Part model, mm, in its own coordinate system. Face numbers are marked on the shaded views. A direction names the side the tool comes from. Give positions to 0.01 mm unless a question says otherwise; leave off trailing zeros. Order: outer loops, then holes, each group sorted by start corner. A loop starts at its lowest first (then second) coordinate and runs counter-clockwise, first axis right, second up.
from build123d import *

# Parameters (mm, degrees)
AUFSATZ_LINEAR_AUSTRAGEN1_DEPTH = 200
AUFSATZ_LINEAR_AUSTRAGEN2_DEPTH = 10
SPIEGELN2_DEPTH                 = 96.337442911
SPIEGELN2_START                 = 104.471237307
SPIEGELN2_2_DEPTH               = 95.528762693
SPIEGELN2_START_2               = 96.337442911
SPIEGELN2_3_DEPTH               = 8.133794396


with BuildPart() as part:
    # Skizze1 → Aufsatz-Linear austragen1 (new body)
    with BuildSketch(Plane.XY):
        with BuildLine():
            Line((0, 38), (-1.4223e-13, 597.0183631567951))
            Line((-1.4223e-13, 597.0183631567951), (125, 597.0183631567951))
            Line((125, 597.0183631567951), (125, 183.98587038126252))
            Line((125, 183.98587038126252), (25.100000000000005, 10.953994705129267))
            ThreePointArc((25.100000000000005, 10.953994705129267), (19.930243299860727, 6.526867548832285), (18.000000000000007, -3.47e-15))
            Line((18.000000000000007, -3.47e-15), (18.000000000000007, -75))
            Line((18.000000000000007, -75), (0, -75))
            Line((0, -75), (0, -38.000000000000014))
            Line((0, -38.000000000000014), (10.000000000000002, -23.000000000000014))
            Line((10.000000000000002, -23.000000000000014), (10.000000000000007, -1.388e-14))
            Line((10.000000000000007, -1.388e-14), (10.000000000000002, 22.999999999999986))
            Line((10.000000000000002, 22.999999999999986), (0, 38))
        make_face()
    extrude(amount=AUFSATZ_LINEAR_AUSTRAGEN1_DEPTH)

    # Skizze2 → Aufsatz-Linear austragen2 (add)
    with BuildSketch(Plane(origin=(0, 597.0183631567951, 0), x_dir=(1, 0, 0), z_dir=(0, 1, 0))):
        Polygon((-1.4223e-13, -200), (35.99999999999986, -200), (35.999999999999865, 0), (1.225e-14, 0), align=None)
    extrude(amount=AUFSATZ_LINEAR_AUSTRAGEN2_DEPTH)

    # Skizze3 → Schnitt-Rotation1 (revolve, cut)
    with BuildSketch(Plane(origin=(0, 0, 0), x_dir=(0, 0, -1), z_dir=(1, 0, 0))):
        Polygon((-105.00000000000001, 72.00000000000001), (-107.50000000000001, 69.5), (-107.50000000000001, 0), (-100, 0), (-100, 72.00000000000001), (-100, 74.88675134594817), align=None)
    revolve(axis=Axis((0, 0, 100), (0, 1, 0)), mode=Mode.SUBTRACT)

    # Spiegeln2: read off the stored shape, not the designer's step
    # Spiegeln2 outline → Spiegeln2 (add)
    with BuildSketch(Plane.XY):
        with BuildLine():
            Line((-36, 607.018363157), (-36, 597.018363157))
            Line((-36, 597.018363157), (-125, 597.018363157))
            Line((-125, 597.018363157), (-125, 183.985870381))
            Line((-125, 183.985870381), (-25.1, 10.953994705))
            ThreePointArc((-25.1, 10.953994705), (-19.9302433, 6.526867549), (-18, 0))
            Line((-18, 0), (-18, -75))
            Line((-18, -75), (0, -75))
            Line((0, -75), (0, -38))
            Line((0, -38), (-10, -23))
            Line((-10, -23), (-10, 23))
            Line((-10, 23), (0, 38))
            Line((0, 38), (0, 607.018363157))
            Line((0, 607.018363157), (-36, 607.018363157))
        make_face()
    extrude(amount=SPIEGELN2_DEPTH)

    # Spiegeln2 2 outline → Spiegeln2 2 (add)
    with BuildSketch(Plane.XY.offset(SPIEGELN2_START)):
        with BuildLine():
            Line((-36, 607.018363157), (-36, 597.018363157))
            Line((-36, 597.018363157), (-125, 597.018363157))
            Line((-125, 597.018363157), (-125, 183.985870381))
            Line((-125, 183.985870381), (-25.1, 10.953994705))
            ThreePointArc((-25.1, 10.953994705), (-19.9302433, 6.526867549), (-18, 0))
            Line((-18, 0), (-18, -75))
            Line((-18, -75), (0, -75))
            Line((0, -75), (0, -38))
            Line((0, -38), (-10, -23))
            Line((-10, -23), (-10, 23))
            Line((-10, 23), (0, 38))
            Line((0, 38), (0, 607.018363157))
            Line((0, 607.018363157), (-36, 607.018363157))
        make_face()
    extrude(amount=SPIEGELN2_2_DEPTH)

    # Spiegeln2 3 outline → Spiegeln2 3 (add)
    with BuildSketch(Plane.XY.offset(SPIEGELN2_START_2)):
        with BuildLine():
            Line((-36, 607.018363157), (-36, 597.018363157))
            Line((-36, 597.018363157), (-125, 597.018363157))
            Line((-125, 597.018363157), (-125, 183.985870381))
            Line((-125, 183.985870381), (-25.1, 10.953994705))
            ThreePointArc((-25.1, 10.953994705), (-19.9302433, 6.526867549), (-18, 0))
            Line((-18, 0), (-18, -75))
            Line((-18, -75), (0, -75))
            Line((0, -75), (0, -38))
            Line((0, -38), (-10, -23))
            Line((-10, -23), (-10, 23))
            Line((-10, 23), (0, 38))
            Line((0, 38), (0, 607.018363157))
            Line((0, 607.018363157), (-36, 607.018363157))
        make_face()
    extrude(amount=SPIEGELN2_3_DEPTH)

    # Spiegeln2 4 outline → Spiegeln2 4 (revolve, cut)
    with BuildSketch(Plane.XY.offset(100)):
        Polygon((5, 72), (0, 74.886751346), (0, 26.711700462), (7.5, 26.711700462), (7.5, 69.5), align=None)
    revolve(axis=Axis((0, 0, 100), (0, 1, 0)), mode=Mode.SUBTRACT)


solid = part.part
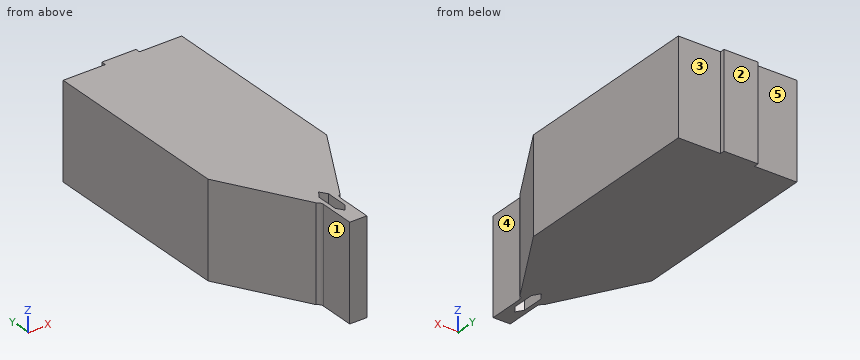
Item 1: Band-saw the part on B-B on x = 83.5. List the corners of the cut face in (y, z), plus the area to 3 significant figures.
Item 2: Band-saw the part on C-C on x = -77. List the corners of the cut face in (y, z), plus the area to 3 significant figures.
Item 3: Drop flat-ended pins along their axis: P1, Ø6, axis at y = 68, z = 109.5, coming from the -X side; P2, Ø14, axis at y = 0.5, z = 89, coming from the +X side; P3, Ø22.5, axis at y = -42.5, z = 72.5, coming from the -X side. Give the stop position or say it passes through.
Item 4: Band-saw the part on A-A on z = 134.5. List the corners of the cut face in (x, y), plus the area to 3 significant figures.
Item 5: Which spindle directions (+Z, -Z, +X, -X, +Y, -Y) get a long thin tool onto all of the face, cutting with end or side? Do the marked faces 1, 2, 3, 4 and 5. Say none if no direction does.
Item 6: Drill centre lines: probe 1 along Z at (x, y) = (0, 41); probe 2 along X at (y, z) = (-19.5, 150.5); probe 3 along Y at (x, z) = (-3.5, 29). Where is each one in solid material? Low to high.
Working result:
1. outline: (112.11, 0) - (597.02, 0) - (597.02, 200) - (112.11, 200) - close
1. area: 97,000 mm2
2. outline: (100.85, 0) - (597.02, 0) - (597.02, 200) - (100.85, 200) - close
2. area: 99,200 mm2
3. P1: stops at x = -59.77
3. P2: stops at x = 20.63
3. P3: stops at x = -18
4. outline: (-125, 183.99) - (-25.1, 10.95) arc R12 cw to (-18, 0) - (-18, -75) - (18, -75) - (18, 0) arc R12 cw to (25.1, 10.95) - (125, 183.99) - (125, 597.02) - (36, 597.02) - (36, 607.02) - (-36, 607.02) - (-36, 597.02) - (-125, 597.02) - close; hole (-10, -23) - (0, -38) - (10, -23) - (10, 23) - (0, 38) - (-10, 23) - close
4. area: 132,000 mm2
5. face 1: +Z, -Z, -X, -Y
5. face 2: +Z, -Z, +X, -X, +Y
5. face 3: +Z, -Z, +X, +Y
5. face 4: +Z, -Z, +X, -Y
5. face 5: +Z, -Z, -X, +Y
6. probe 1: z = 0 to 92.5, 107.5 to 200
6. probe 2: x = -18 to -10, 10 to 18
6. probe 3: y = -75 to -32.75, 32.75 to 607.02
